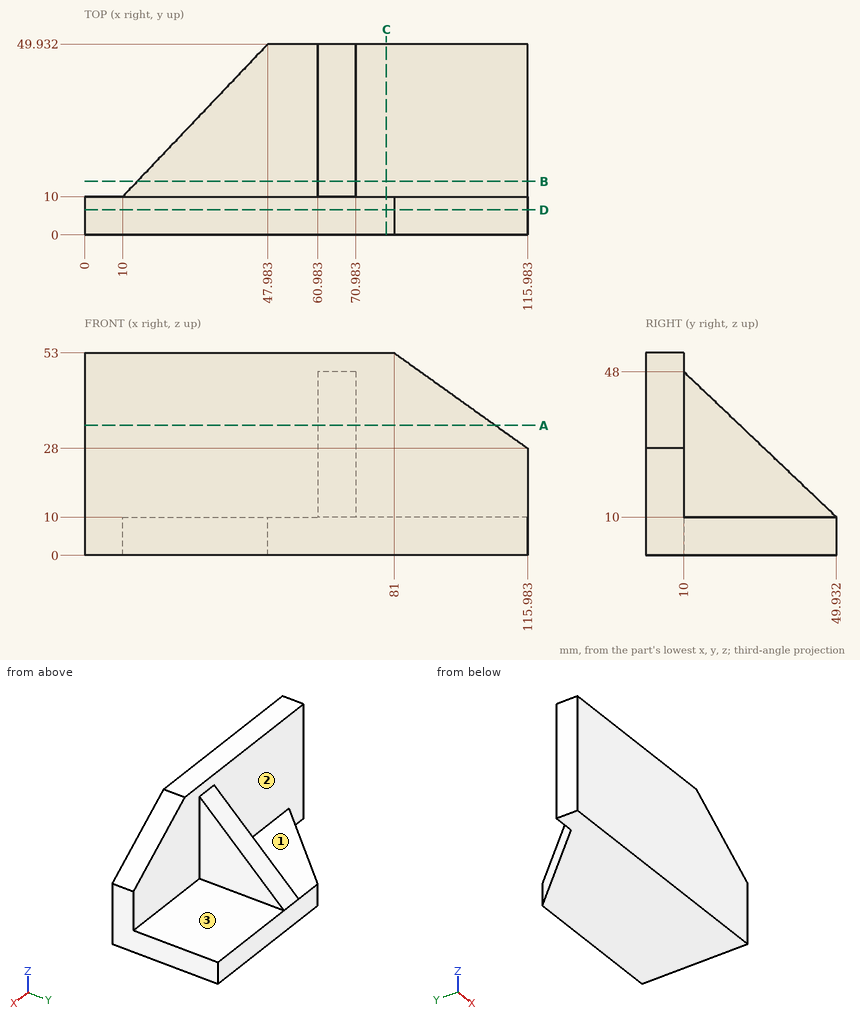
The figure shows three views and two pictorial views of one solid part (mm, origin at its lowest corner). Answer the questions. A direction names the side the tool comes from. Give positions to 0.01 mm unless a question says otherwise; leave off trailing zeros. Order: outer loops, then holes, each group sorted by start corner. A loop starts at its lowest first (then second) coordinate and runs counter-clockwise, first axis right, second up. Notation, with made-up numbers: M 0.5,54.25 L 55.5,54.25 A25 cw 55.5,76.25 Z; hole C -5.75,55.25 d7. An arc over 180 degrees is marked long. Return JSON: item names as keys, results as strings.
1) Section A-A, the plane z = 34 is taken. Write down the section's boundary in (x, y), plus the area to 3 significant figures.
Resolved:
{"outline": "M 0,0 L 107.59,0 L 107.59,10 L 70.98,10 L 70.98,24.71 L 60.98,24.71 L 60.98,10 L 0,10 Z", "area": "1,220 mm^2"}
2) Section B-B, the plane y = 14 is taken. Write down the section's boundary in (x, z) (1 decimal), plus the area to 3 significant figures.
Resolved:
{"outline": "M 13.8,0 L 116,0 L 116,10 L 71,10 L 71,44.2 L 61,44.2 L 61,10 L 13.8,10 Z", "area": "1,360 mm^2"}
3) Section C-C, the plane x = 79 is taken. Write down the section's boundary in (y, z).
Resolved:
{"outline": "M 0,0 L 49.93,0 L 49.93,10 L 10,10 L 10,53 L 0,53 Z"}
4) Each of these flat-tipped pins is pushed along its axis until it touches: pin 1 (1.5 mm diameter, centred on y = 16, z = 13, fed in from +X); pin 2 (12 mm diameter, centred on x = 23.5, y = 25.5, fed in from +Z); pin 3 (5 mm diameter, centred on y = 23, z = 27.5, fed in from -X). Where does it stop, or does it pass through?
Resolved:
{"pin 1": "x = 70.98", "pin 2": "z = 10", "pin 3": "x = 60.98"}
5) Section D-D, the plane y = 6.5 is taken. Write down the section's boundary in (x, z), plus the area to 3 significant figures.
Resolved:
{"outline": "M 0,0 L 115.98,0 L 115.98,28 L 81,53 L 0,53 Z", "area": "5,710 mm^2"}
6) Straight lines are drawn through the part: line 1 along Z through (x, y) = (91, 41.5); line 2 along X through (y, z) = (10.5, 18.5). For each, find the intervals that lie inside material, in ascending order. Write a range as [from, to].
Resolved:
{"line 1": "[0, 10]", "line 2": "[60.98, 70.98]"}
7) A tool of negligible diameter and unlimited length cuts with its end or side. For the marked faces 1, 2 and 3, from which of +Z, -Z, +X, -X, +Y, -Y can it reach the whole face along a straight path? Write none if from no direction.
Resolved:
{"face 1": "+Z, -X, +Y", "face 2": "+Z, +Y", "face 3": "+Z, +X, +Y"}
